Read the model definition and answer for the solid it produces. Units are mm, in the model's axes. Face numbers are marked on the shaded views. A direction names the side the tool comes from. Round coordinates to 2 decimals unless told otherwise and drop trailing zeros. Order: outer loops, then holes, each group sorted by start corner. A loop starts at its lowest first (then second) coordinate and runs counter-clockwise, first axis right, second up.
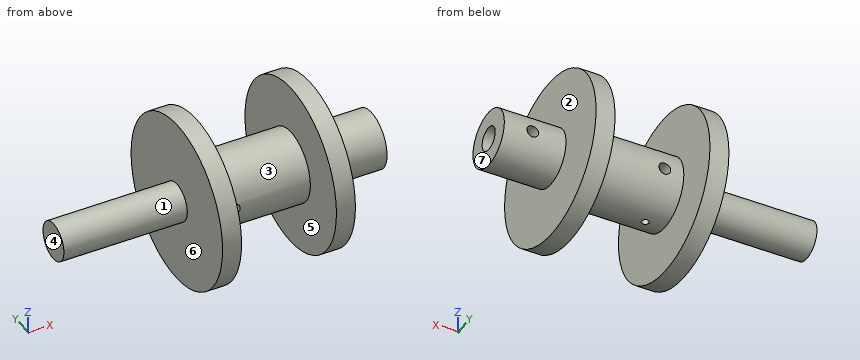
Autodesk Inventor part; units mm, degrees
ref_plane "Arbeitsebene1" through (0, 0, 7.5) normal (0, 0, 1) x (1, 0, 0)
ref_plane "Arbeitsebene2" through (0, -7.5, 0) normal (0, 1, 0) x (-1, 0, 0)
ref_plane "Arbeitsebene3" through (20.5, 6, 0) normal (0, 1, 0) x (-1, 0, 0)
sketch "Skizze1" plane through (0, 0, 0) normal (0, 0, 1) x (1, 0, 0)
  line L0 (-53.4, 0) -> (40.4, 0)
  line L1 (0, -3.5) -> (0, 21)
  line L2 (-10, 7.5) -> (10, 7.5)
  line L3 (10, 7.5) -> (10, 17.5)
  line L4 (10, 17.5) -> (14, 17.5)
  line L5 (14, 17.5) -> (14, 6)
  line L6 (14, 6) -> (27, 6)
  line L7 (27, 6) -> (27, 0)
  line L8 (-10, 7.5) -> (-10, 17.5)
  line L9 (-10, 17.5) -> (-14, 17.5)
  line L10 (-14, 17.5) -> (-14, 4)
  line L11 (-14, 4) -> (-40, 4)
  line L12 (-40, 4) -> (-40, 0)
  line L13 (-40, 0) -> (27, 0)
  point P0 (0, 0)
  dimension "d0" = 20
  dimension "d1" = 15
  dimension "d2" = 28
  dimension "d3" = 10
  dimension "d4" = 8
  dimension "d5" = 40
  dimension "d6" = 12
  dimension "d7" = 27
revolve "Umdrehung1" add sketch "Skizze1" angle 360 about axis through (-40, 0, 0) along (1, 0, 0)
ref_plane "Arbeitsebene1" through (0, 0, 7.5) normal (0, 0, 1) x (1, 0, 0)
ref_plane "Arbeitsebene2" through (0, -7.5, 0) normal (0, 1, 0) x (-1, 0, 0)
sketch "Skizze2" plane through (0, 0, 7.5) normal (0, 0, 1) x (1, 0, 0)
  line L0 (-53.4, 0) -> (40.4, 0)
  line L1 (0, -24.5) -> (0, 24.5)
  point P0 (0, 0)
  point P1 (-6, 0)
  dimension "d9" = 6
hole "Bohrung1" at (-6, 0, 7.5) direction (0, 0, -1) diameter 1.5 end through all
sketch "Skizze3" plane through (0, -7.5, 0) normal (0, 1, 0) x (-1, 0, 0)
  line L0 (53.4, 0) -> (-40.4, 0)
  line L1 (0, -24.5) -> (0, 24.5)
  point P0 (0, 0)
  point P1 (6, 0)
  dimension "d17" = 6
hole "Bohrung2" at (-6, -7.5, 0) direction (0, 1, 0) diameter 2.459 end through all
hole "Bohrung3" at (27, 0, 0) direction (-1, 0, 0) diameter 5 depth 25 tip angle 118
ref_plane "Arbeitsebene3" through (20.5, 6, 0) normal (0, 1, 0) x (-1, 0, 0)
sketch "Skizze6" plane through (20.5, 6, 0) normal (0, 1, 0) x (-1, 0, 0)
  line L0 (-6.5, 6) -> (-6.5, -6)
  line L1 (73.9, 0) -> (-19.9, 0)
  line L2 (20.5, -24.5) -> (20.5, 24.5)
  point P0 (20.5, 0)
  point P1 (-0.5, 0)
  dimension "d36" = 6
hole "Bohrung4" at (21, 6, 0) direction (0, -1, 0) diameter 2.459 end up to surface
properties part number "13_0204_055"
Q1. A cutting plane is placed at D-D, the plane x = -32. Give the vertices of the cut face in (y, z).
Outcome:
outline: circle Ø8 at (0, 0)
Q2. Flat-ended cylindrical pins translate along their axes: pin 1 (2.5 mm diameter, centred on x = -6, y = 0, fed in from +Z); pin 2 (1 mm diameter, centred on x = 2.5, y = -4.5, fed in from +Z); pin 3 (3 mm diameter, centred on y = 12, z = -4.5, fed in from +X); pin 4 (1.4 mm diameter, centred on x = -6, y = 0, fed in from +Z). Find the tip coordinate at first contact, or state that the pin passes through.
Outcome:
pin 1: stops at z = 7.5
pin 2: stops at z = 6.34
pin 3: stops at x = 14
pin 4: passes through
Q3. A cutting plane is placed at B-B, the plane x = -6. Give the vertices of the cut face in (y, z).
Outcome:
outline: (-7.4, -1.23) arc R7.5 ccw to (-0.75, -7.46) - (-0.75, -1.23) - close; (-7.4, 1.23) - (-0.75, 1.23) - (-0.75, 7.46) arc R7.5 ccw to start; (0.75, -7.46) arc R7.5 ccw to (7.4, -1.23) - (0.75, -1.23) - close; (0.75, 1.23) - (7.4, 1.23) arc R7.5 ccw to (0.75, 7.46) - close
Q4. A cutting plane is placed at A-A, the plane z = -12. Give the vertices of the cut face in (x, y), plus the area to 3 significant figures.
Outcome:
outline: (-14, -12.74) - (-10, -12.74) - (-10, 12.74) - (-14, 12.74) - close; (10, -12.74) - (14, -12.74) - (14, 12.74) - (10, 12.74) - close
area: 204 mm2
Q5. For a pull along X with two mould halves and no side action, classify the marked faces 5, 6 and 7 as released by +X, released by -X, zero draft, split by the parting line, or undercut.
Outcome:
face 5: undercut
face 6: released by -X
face 7: released by +X
Q6. Straight lines are drawn through the part: probe 1 along Z at (x, y) = (8, 0); probe 2 along X at (y, z) = (5, -8.5); probe 3 along Z at (x, y) = (-5, -5). For each, find the intervals that lie inside material, in ascending order.
Outcome:
probe 1: z = -7.5 to -2.5, 2.5 to 7.5
probe 2: x = -14 to -10, 10 to 14
probe 3: z = -5.59 to -0.72, 0.72 to 5.59
Q7. A cutting plane is placed at C-C, the plane y = -10. Give the vertices of the cut face in (x, z), plus the area to 3 significant figures.
Outcome:
outline: (-14, -14.36) - (-10, -14.36) - (-10, 14.36) - (-14, 14.36) - close; (10, -14.36) - (14, -14.36) - (14, 14.36) - (10, 14.36) - close
area: 230 mm2
Q8. For the marked faces 1, 2, 3 and 4, determine the directions among +Z, -Z, +X, -X, +Y, -Y from which every point of the face is accessible in a straight line to the end or side of a thin tool.
Outcome:
face 1: -X
face 2: +X
face 3: none
face 4: +Z, -Z, -X, +Y, -Y
